```python
from build123d import *

# Parameters (mm, degrees)
BOSS_EXTRUDE1_DEPTH = 31.6
SKETCH4_W           = 12.7
SKETCH4_H           = 10
SKETCH4_W_2         = 8.3
SKETCH4_H_2         = 7.8
SKETCH4_W_3         = 5.8
SKETCH4_H_3         = 7.6
BOSS_EXTRUDE2_DEPTH = 0.35
FILLET1_R           = 0.5
SKETCH5_R           = 0.25
BOSS_EXTRUDE3_DEPTH = 0.1
SKETCH19_W          = 17.3
SKETCH19_H          = 2.2
CUT_EXTRUDE11_DEPTH = 36.553470936
FILLET2_R           = 0.5
SKETCH21_W          = 0.1
SKETCH21_H          = 9.7
CUT_EXTRUDE13_DEPTH = 0.1
SKETCH20_W          = 5.5
SKETCH20_H          = 7.5
CUT_EXTRUDE12_DEPTH = 36.945875479
SKETCH22_W          = 7.3
SKETCH22_H          = 12.7
CUT_EXTRUDE14_DEPTH = 11.3
SKETCH22_3_W        = 7.3
SKETCH22_3_H        = 7.4
SKETCH22_3_H_2      = 6.5
CUT_EXTRUDE15_DEPTH = 9.1
SKETCH23_W          = 6.5
SKETCH23_H          = 8.6
CUT_EXTRUDE16_DEPTH = 0.7
BOSS_EXTRUDE4_REACH = 37.07


with BuildPart() as part:
    # Sketch2 → Boss-Extrude1 (new body)
    with BuildSketch(Plane.XY):
        with BuildLine():
            Line((-0.965868705, -13.448021996), (-0.965868705, -8.948021996))
            ThreePointArc((-0.965868705, -8.948021996), (-6.152703888, -6.568427123), (-8.865868705, -1.548021996))
            Line((-8.865868705, -1.548021996), (-10.165868705, -1.548021996))
            Line((-10.165868705, -1.548021996), (-10.165868705, -13.448021996))
            Line((-10.165868705, -13.448021996), (-0.965868705, -13.448021996))
        make_face()
    extrude(amount=-BOSS_EXTRUDE1_DEPTH)

    # Sketch4 → Boss-Extrude2 (add)
    with BuildSketch(Plane.ZY.offset(10.165868705)):
        with Locations((-7.15, -7.248021996)):
            Rectangle(SKETCH4_W, SKETCH4_H)
        with Locations((-19.35, -6.148021996)):
            Rectangle(SKETCH4_W_2, SKETCH4_H_2)
        with Locations((-28.1, -6.048021996)):
            Rectangle(SKETCH4_W_3, SKETCH4_H_3)
    extrude(amount=BOSS_EXTRUDE2_DEPTH)

    # Fillet1
    fillet1_edges = [part.edges().sort_by_distance(p)[0] for p in [
        (-10.340868705, -2.248021996, -13.5),
        (-10.340868705, -12.248021996, -13.5),
        (-10.340868705, -12.248021996, -0.8),
        (-10.340868705, -2.248021996, -0.8),
        (-10.340868705, -2.248021996, -31),
        (-10.340868705, -9.848021996, -31),
        (-10.340868705, -9.848021996, -25.2),
        (-10.340868705, -2.248021996, -25.2),
        (-10.340868705, -2.248021996, -23.5),
        (-10.340868705, -10.048021996, -23.5),
        (-10.340868705, -10.048021996, -15.2),
        (-10.340868705, -2.248021996, -15.2),
    ]]
    fillet(fillet1_edges, radius=FILLET1_R)

    # Sketch5 → Boss-Extrude3 (add)
    with BuildSketch(Plane.ZY.offset(10.515868705)):
        with Locations(Location((-13, -2.748021996, 0), (0, 0, 180))):
            Circle(SKETCH5_R)
        with Locations(Location((-1.3, -2.748021996, 0), (0, 0, 180))):
            Circle(SKETCH5_R)
        with Locations((-23, -2.748021996)):
            Circle(SKETCH5_R)
        with Locations((-23, -9.548021996)):
            Circle(SKETCH5_R)
        with Locations(Location((-1.3, -11.748021996, 0), (0, 0, 180))):
            Circle(SKETCH5_R)
        with Locations(Location((-13, -11.748021996, 0), (0, 0, 180))):
            Circle(SKETCH5_R)
        with Locations((-15.7, -2.748021996)):
            Circle(SKETCH5_R)
        with Locations((-15.7, -9.548021996)):
            Circle(SKETCH5_R)
        with Locations((-30.5, -2.748021996)):
            Circle(SKETCH5_R)
        with Locations((-25.7, -2.748021996)):
            Circle(SKETCH5_R)
        with Locations((-25.7, -9.348021996)):
            Circle(SKETCH5_R)
        with Locations((-30.5, -9.348021996)):
            Circle(SKETCH5_R)
    extrude(amount=BOSS_EXTRUDE3_DEPTH)

    # Sketch19 → Cut-Extrude11 (cut, through all)
    with BuildSketch(Plane.ZY.offset(10.165868705)):
        with Locations((-22.95, -12.348021996)):
            Rectangle(SKETCH19_W, SKETCH19_H)
    extrude(amount=-CUT_EXTRUDE11_DEPTH, mode=Mode.SUBTRACT)

    # Fillet2
    fillet2_edges = [part.edges().sort_by_distance(p)[0] for p in [
        (-10.165868705, -13.448021996, -7.15),
        (-10.165868705, -11.248021996, -22.95),
    ]]
    fillet(fillet2_edges, radius=FILLET2_R)

    # Sketch21 → Cut-Extrude13 (cut)
    with BuildSketch(Plane.ZY.offset(10.165868705)):
        with Locations((-14.35, -6.398021996)):
            Rectangle(SKETCH21_W, SKETCH21_H)
        with Locations((-24.35, -6.398021996)):
            Rectangle(SKETCH21_W, SKETCH21_H)
    extrude(amount=-CUT_EXTRUDE13_DEPTH, mode=Mode.SUBTRACT)

    # Sketch20 → Cut-Extrude12 (cut, through all)
    with BuildSketch(Plane(origin=(0, 0, 0), x_dir=(1, 0, 0), z_dir=(0, 1, 0))):
        with Locations((-3.715868705, 12.25)):
            Rectangle(SKETCH20_W, SKETCH20_H)
    extrude(amount=-CUT_EXTRUDE12_DEPTH, mode=Mode.SUBTRACT)

    # Sketch22 → Cut-Extrude14 (cut)
    with BuildSketch(Plane(origin=(0, -1.548021996, 0), x_dir=(1, 0, 0), z_dir=(0, 1, 0))):
        with Locations((-5.215868705, 7.35)):
            Rectangle(SKETCH22_W, SKETCH22_H)
    extrude(amount=-CUT_EXTRUDE14_DEPTH, mode=Mode.SUBTRACT)

    # Sketch22<3> → Cut-Extrude15 (cut)
    with BuildSketch(Plane(origin=(0, -1.548021996, 0), x_dir=(1, 0, 0), z_dir=(0, 1, 0))):
        with Locations((-5.215868705, 17.4)):
            Rectangle(SKETCH22_3_W, SKETCH22_3_H)
        with Locations((-5.215868705, 27.35)):
            Rectangle(SKETCH22_3_W, SKETCH22_3_H_2)
    extrude(amount=-CUT_EXTRUDE15_DEPTH, mode=Mode.SUBTRACT)

    # Sketch23 → Cut-Extrude16 (cut)
    with BuildSketch(Plane(origin=(-8.865868705, 0, 0), x_dir=(0, 0, -1), z_dir=(1, 0, 0))):
        Polygon((1, -12.848021996), (13.7, -12.848021996), (13.7, -10.648021996), (21.1, -10.648021996), (21.1, -2.048021996), (1, -2.048021996), align=None)
        with Locations((27.35, -6.348021996)):
            Rectangle(SKETCH23_W, SKETCH23_H)
    extrude(amount=-CUT_EXTRUDE16_DEPTH, mode=Mode.SUBTRACT)

    # Sketch24 → Boss-Extrude4 (add, up to next)
    with BuildSketch(Plane(origin=(0, 0, -1), x_dir=(-1, 0, 0), z_dir=(0, 0, -1)), mode=Mode.PRIVATE) as boss_extrude4_sk1:
        with BuildLine():
            Line((8.865868705, -2.048021996), (8.865868705, -1.548021996))
            ThreePointArc((8.865868705, -1.548021996), (8.818419162, -1.798744975), (8.763880756, -2.048021996))
            Line((8.763880756, -2.048021996), (8.865868705, -2.048021996))
        make_face()
    boss_extrude4_tool1 = extrude(boss_extrude4_sk1.sketch, amount=BOSS_EXTRUDE4_REACH, mode=Mode.PRIVATE) - part.part
    add(boss_extrude4_tool1.solids().sort_by_distance((-8.832663, -1.885567, -1))[0])
    add(boss_extrude4_tool1.solids().sort_by_distance((-8.832663, -1.885567, -1))[1])


solid = part.part
```
Geometry: final body of the model. Coordinates: model frame, mm. A direction names the side the tool comes from. Coordinates: 2 decimals unless noted, no trailing zeros. Order: outer loops, then holes, each group sorted by start corner. A loop starts at its lowest first (then second) coordinate and runs counter-clockwise, first axis right, second up. Notation, with made-up numbers: M 9,-1.75 L 56,-1.75 A27 ccw 56,33.25 Z; hole C -32,84 d8. An arc over 180 degrees is marked long. Answer in a Markdown table with one row per item. Add a question column.
Q1. Reachability of faces 1 (the flat face through (-1.566, -10, -19)), 2 (the flat face through (-10.516, -6, -19)), 3 (the flat face through (-9.566, -7, -11)) from +Z, -Z, +X, -X, +Y, -Y: full face, straight path, thin tool, end or side. Return the list, or none.
Q2. Contact query for flat-ended pins moving along their axis: P1, Ø3, axis at y = -11.5, z = -10.5, coming from the +X side; P2, Ø1.5, axis at y = -4.5, z = -13, coming from the +X side; P3, Ø2, axis at y = -11, z = -11, coming from the -X side; P4, Ø1.1, axis at x = -7.5, y = -11.5, coming from the +Z side. Output: stop coordinate, or through.
Q3. Section query D-D on x = -4.5. Return the cut outline in (y, z).
Q4. Line query: L1, parallel to Z at x = -4, y = -9.75; L2, parallel to Z at x = -9.5, y = -11.75; L3, parallel to X at y = -7.5, z = -15.5. Output: solid intervals per line, ascending.
Q5. Section query B-B on x = -6. Return the cut outline in (y, z), and give its area (3 significant figures).
Q6. Section query A-A on z = -2.5. Return the cut outline in (x, y).
Q7. Mould query, pull axis Z, two halves, no side actions, for faces 4 (the flat face through (-3, -13, -8.5)), 5 (the flat face through (-6, -10.648, -18)), 6 (the flat face through (-7, -9, 0)), 7 (the flat face through (-5, -11.248, -23)). Classes: released by +Z, released by -Z, zero draft, split by the parting line, or undercut.
Completed:
| question | item | result |
|---|---|---|
| 1 | face 1 | +Y |
| 1 | face 2 | -X |
| 1 | face 3 | none |
| 2 | P1 | stops at x = -6.47 |
| 2 | P2 | stops at x = -9.57 |
| 2 | P3 | stops at x = -10.52 |
| 2 | P4 | stops at z = 0 |
| 3 | outline | M -13.45,-8.5 L -12.85,-8.5 L -12.85,-1 L -7.79,-1 L -7.79,0 L -13.45,0 Z; M -11.25,-31.6 L -7.79,-31.6 L -7.79,-30.6 L -10.65,-30.6 L -10.65,-24.1 L -7.79,-24.1 L -7.79,-21.1 L -10.65,-21.1 L -10.65,-16 L -11.25,-16 Z |
| 4 | L1 | z = -31.6 to -30.6, -24.1 to -21.1, -1 to 0 |
| 4 | L2 | z = -14.3 to -13.7, -1 to 0 |
| 4 | L3 | x = -10.52 to -9.57 |
| 5 | outline | M -13.45,-8.5 L -12.85,-8.5 L -12.85,-1 L -6.71,-1 L -6.71,0 L -13.45,0 Z; M -11.25,-31.6 L -6.71,-31.6 L -6.71,-30.6 L -10.65,-30.6 L -10.65,-24.1 L -6.71,-24.1 L -6.71,-21.1 L -10.65,-21.1 L -10.65,-16 L -11.25,-16 Z |
| 5 | area | 36.4 mm2 |
| 6 | outline | M -10.52,-12.25 L -10.17,-12.25 L -10.17,-12.95 A0.5 ccw -9.67,-13.45 L -0.97,-13.45 L -0.97,-8.95 A9 cw -1.57,-8.86 L -1.57,-12.85 L -9.57,-12.85 L -9.57,-2.05 L -8.76,-2.05 A9 cw -8.87,-1.55 L -10.17,-1.55 L -10.17,-2.25 L -10.52,-2.25 Z |
| 7 | face 4 | undercut |
| 7 | face 5 | undercut |
| 7 | face 6 | released by +Z |
| 7 | face 7 | zero draft |
